For this review, take the finished solid that the model builds, in its own axes (mm). Give positions to 0.01 mm unless a question says otherwise; leave off trailing zeros. Write each loop counter-clockwise with the first axis right and the second up, starting at its lowest first coordinate (ties: lowest second). Pieces come first, ordered by that corner, then holes.
Q1. For line 1 (Z direction, x = -143.5, y = 0.75); line 2 (Z direction, x = -147, y = 0.35); line 3 (Z direction, x = -50.5, y = 1.3), list the stretches that pass through material, from the lowest coordinate up.
Q2. We need section B-B (y = 0.5). Give the number of separate pieces and of enclosed holes in the cut face, then the cut area to 3 significant figures.
Q3. We need section A-A (z = 266.5). Write out the cut boundary in (x, y).
Q4. Insertion check: P1, Ø0.5, axis at y = 1, z = 134, coming from the -X side; P2, Ø0.8, axis at y = 0.5, z = 320.5, coming from the +X side. Each pin has a flat end and moves straight along its axis. Give the tip position at first contact, or say it passes through.
Q5. We need section C-C (z = 183). Write out the cut boundary in (x, y).
```python
from build123d import *

# Parameters (mm, degrees)
SKETCH1_R        = 1.85915493
SKETCH1_R_2      = 2
SKETCH1_R_3      = 1.28892694
SKETCH1_R_4      = 1.407234354
SKETCH1_R_5      = 1.5
SKETCH1_R_6      = 1.673239437
EXTRUSION1_DEPTH = 1.6
FILLET1_R        = 1
FILLET2_R        = 4
FILLET3_R        = 3
FILLET4_R        = 3
FILLET5_R        = 2
FILLET6_R        = 2
FILLET7_R        = 3
FILLET8_R        = 3
FILLET9_R        = 2
FILLET10_R       = 2
FILLET11_R       = 3


with BuildPart() as part:
    # Sketch1 → Extrusion1 (new body)
    with BuildSketch(Plane(origin=(0, 0, 0), x_dir=(-1, 0, 0), z_dir=(0, 1, 0))):
        Polygon((74.087520418, 321.088295015), (70.369210559, 327.285477572), (45.580478165, 327.285477572), (45.580478165, 312.412238135), (23.246043749, 290.934342561), (26.682507041, 287.360833055), (12.735407819, 253.538985229), (9.017097883, 253.538985229), (9.017097883, 226.891111382), (9.017097883, 200.243237534), (12.735407819, 200.243237534), (26.682507041, 166.421389708), (23.246043749, 162.847880202), (45.580478165, 141.369984628), (45.580478165, 126.496745191), (70.369210559, 126.496745191), (74.087520418, 132.693927748), (97.636816193, 132.693927748), (121.186111968, 132.693927748), (124.904421827, 126.496745191), (149.693154221, 126.496745191), (149.693154221, 141.369984628), (172.027588636, 162.847880202), (168.591125345, 166.421389708), (182.538224567, 200.243237534), (186.256534503, 200.243237534), (186.256534503, 226.891111382), (186.256534503, 253.538985229), (182.538224567, 253.538985229), (168.591125345, 287.360833055), (172.027588636, 290.934342561), (149.693154221, 312.412238135), (149.693154221, 327.285477572), (124.904421827, 327.285477572), (121.186111968, 321.088295015), (97.636816193, 321.088295015), align=None)
        with Locations((49.266182018, 151.62213525)):
            Circle(SKETCH1_R, mode=Mode.SUBTRACT)
        with Locations((117.636816193, 226.891111382)):
            Circle(SKETCH1_R_2, mode=Mode.SUBTRACT)
        with Locations((77.636816193, 226.891111382)):
            Circle(SKETCH1_R_2, mode=Mode.SUBTRACT)
        with Locations((97.636816193, 226.891111382)):
            Circle(SKETCH1_R_2, mode=Mode.SUBTRACT)
        with Locations((12.517097883, 215.891111382)):
            Circle(SKETCH1_R_3, mode=Mode.SUBTRACT)
        with Locations((12.517097883, 237.891111382)):
            Circle(SKETCH1_R_4, mode=Mode.SUBTRACT)
        with Locations((107.636816193, 316.338295015)):
            Circle(SKETCH1_R_5, mode=Mode.SUBTRACT)
        with Locations((87.636816193, 316.338295015)):
            Circle(SKETCH1_R_5, mode=Mode.SUBTRACT)
        with Locations((87.636816193, 137.443927748)):
            Circle(SKETCH1_R_5, mode=Mode.SUBTRACT)
        with Locations((107.636816193, 137.443927748)):
            Circle(SKETCH1_R_5, mode=Mode.SUBTRACT)
        with Locations((182.756534503, 215.891111382)):
            Circle(SKETCH1_R_3, mode=Mode.SUBTRACT)
        with Locations((182.756534503, 237.891111382)):
            Circle(SKETCH1_R_4, mode=Mode.SUBTRACT)
        with Locations((176.256534503, 235.141111382)):
            Circle(SKETCH1_R_6, mode=Mode.SUBTRACT)
        with Locations((176.256534503, 218.641111382)):
            Circle(SKETCH1_R_6, mode=Mode.SUBTRACT)
        with Locations((51.777661187, 316.130534525)):
            Circle(SKETCH1_R, mode=Mode.SUBTRACT)
        with Locations((49.266182018, 302.160087513)):
            Circle(SKETCH1_R, mode=Mode.SUBTRACT)
        with Locations((19.017097883, 235.141111382)):
            Circle(SKETCH1_R_6, mode=Mode.SUBTRACT)
        with Locations((143.495971199, 137.651688238)):
            Circle(SKETCH1_R, mode=Mode.SUBTRACT)
        with Locations((146.007450368, 151.62213525)):
            Circle(SKETCH1_R, mode=Mode.SUBTRACT)
        with Locations((143.495971199, 316.130534525)):
            Circle(SKETCH1_R, mode=Mode.SUBTRACT)
        with Locations((146.007450368, 302.160087513)):
            Circle(SKETCH1_R, mode=Mode.SUBTRACT)
        with Locations((19.017097883, 218.641111382)):
            Circle(SKETCH1_R_6, mode=Mode.SUBTRACT)
        with Locations((51.777661187, 137.651688238)):
            Circle(SKETCH1_R, mode=Mode.SUBTRACT)
        with Locations((42.888078851, 158.000238416)):
            Circle(SKETCH1_R, mode=Mode.SUBTRACT)
        with Locations((152.385553534, 295.781984347)):
            Circle(SKETCH1_R, mode=Mode.SUBTRACT)
        with Locations((42.888078851, 295.781984347)):
            Circle(SKETCH1_R, mode=Mode.SUBTRACT)
        with Locations((152.385553534, 158.000238416)):
            Circle(SKETCH1_R, mode=Mode.SUBTRACT)
    extrude(amount=EXTRUSION1_DEPTH)

    # Fillet1
    fillet1_edges = [part.edges().sort_by_distance(p)[0] for p in [
        (-121.186111968, 0.8, 321.088295015),
        (-121.186111968, 0.8, 132.693927748),
        (-74.087520418, 0.8, 132.693927748),
        (-74.087520418, 0.8, 321.088295015),
    ]]
    fillet(fillet1_edges, radius=FILLET1_R)

    # Fillet2
    fillet2_edges = [part.edges().sort_by_distance(p)[0] for p in [
        (-149.693154221, 0.8, 327.285477572),
        (-149.693154221, 0.8, 126.496745191),
        (-45.580478165, 0.8, 126.496745191),
        (-45.580478165, 0.8, 327.285477572),
    ]]
    fillet(fillet2_edges, radius=FILLET2_R)

    # Fillet3
    fillet3_edges = [part.edges().sort_by_distance(p)[0] for p in [
        (-149.693154221, 0.8, 312.412238135),
        (-149.693154221, 0.8, 141.369984628),
        (-45.580478165, 0.8, 141.369984628),
        (-45.580478165, 0.8, 312.412238135),
    ]]
    fillet(fillet3_edges, radius=FILLET3_R)

    # Fillet4
    fillet4_edges = [part.edges().sort_by_distance(p)[0] for p in [
        (-172.027588636, 0.8, 290.934342561),
    ]]
    fillet(fillet4_edges, radius=FILLET4_R)

    # Fillet5
    fillet5_edges = [part.edges().sort_by_distance(p)[0] for p in [
        (-168.591125345, 0.8, 287.360833055),
    ]]
    fillet(fillet5_edges, radius=FILLET5_R)

    # Fillet6
    fillet6_edges = [part.edges().sort_by_distance(p)[0] for p in [
        (-26.682507041, 0.8, 287.360833055),
    ]]
    fillet(fillet6_edges, radius=FILLET6_R)

    # Fillet7
    fillet7_edges = [part.edges().sort_by_distance(p)[0] for p in [
        (-23.246043749, 0.8, 290.934342561),
    ]]
    fillet(fillet7_edges, radius=FILLET7_R)

    # Fillet8
    fillet8_edges = [part.edges().sort_by_distance(p)[0] for p in [
        (-172.027588636, 0.8, 162.847880202),
        (-23.246043749, 0.8, 162.847880202),
    ]]
    fillet(fillet8_edges, radius=FILLET8_R)

    # Fillet9
    fillet9_edges = [part.edges().sort_by_distance(p)[0] for p in [
        (-168.591125345, 0.8, 166.421389708),
        (-26.682507041, 0.8, 166.421389708),
    ]]
    fillet(fillet9_edges, radius=FILLET9_R)

    # Fillet10
    fillet10_edges = [part.edges().sort_by_distance(p)[0] for p in [
        (-182.538224567, 0.8, 253.538985229),
        (-182.538224567, 0.8, 200.243237534),
        (-12.735407819, 0.8, 200.243237534),
        (-12.735407819, 0.8, 253.538985229),
    ]]
    fillet(fillet10_edges, radius=FILLET10_R)

    # Fillet11
    fillet11_edges = [part.edges().sort_by_distance(p)[0] for p in [
        (-186.256534503, 0.8, 200.243237534),
        (-186.256534503, 0.8, 253.538985229),
        (-9.017097883, 0.8, 253.538985229),
        (-9.017097883, 0.8, 200.243237534),
    ]]
    fillet(fillet11_edges, radius=FILLET11_R)


solid = part.part
```
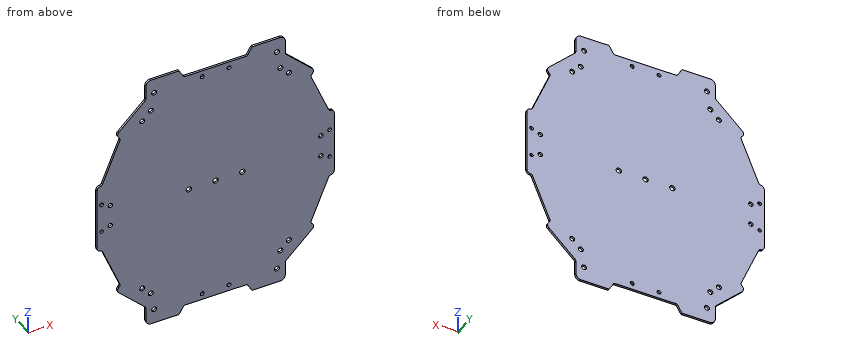
Computed:
1. line 1: z = 126.5 to 135.79, 139.51 to 314.27, 317.99 to 327.29
1. line 2: z = 126.72 to 150.05, 153.19 to 300.59, 303.73 to 327.07
1. line 3: z = 126.5 to 136.3, 139 to 150.23, 153.01 to 300.77, 303.55 to 314.78, 317.48 to 327.29
2. separate pieces: 1
2. enclosed holes: 27
2. area: 28,600 mm2
3. outline: (-177.19, 0) - (-18.08, 0) - (-18.08, 1.6) - (-177.19, 1.6) - close
4. P1: stops at x = -149.69
4. P2: stops at x = -45.58
5. outline: (-175.43, 0) - (-19.85, 0) - (-19.85, 1.6) - (-175.43, 1.6) - close
